Study the drawing (mm; zero at the part's minimum x, y, z) and answer. Coordinates: 2 decimals unless noted, no trailing zeros. Loops run counter-clockwise (first coordinate to the right, second up) from the corner with the lowest first, then second, coordinate; pieces in that order, holes last. Notation, with made-up numbers: (-9, 88.5) -> (4, 88.5) arc R14 cw to (4, 106.5) -> close; hole circle Ø5 at (59, 53.5). An arc over 180 degrees is marked (long way). Answer in a Markdown table with one row per item.
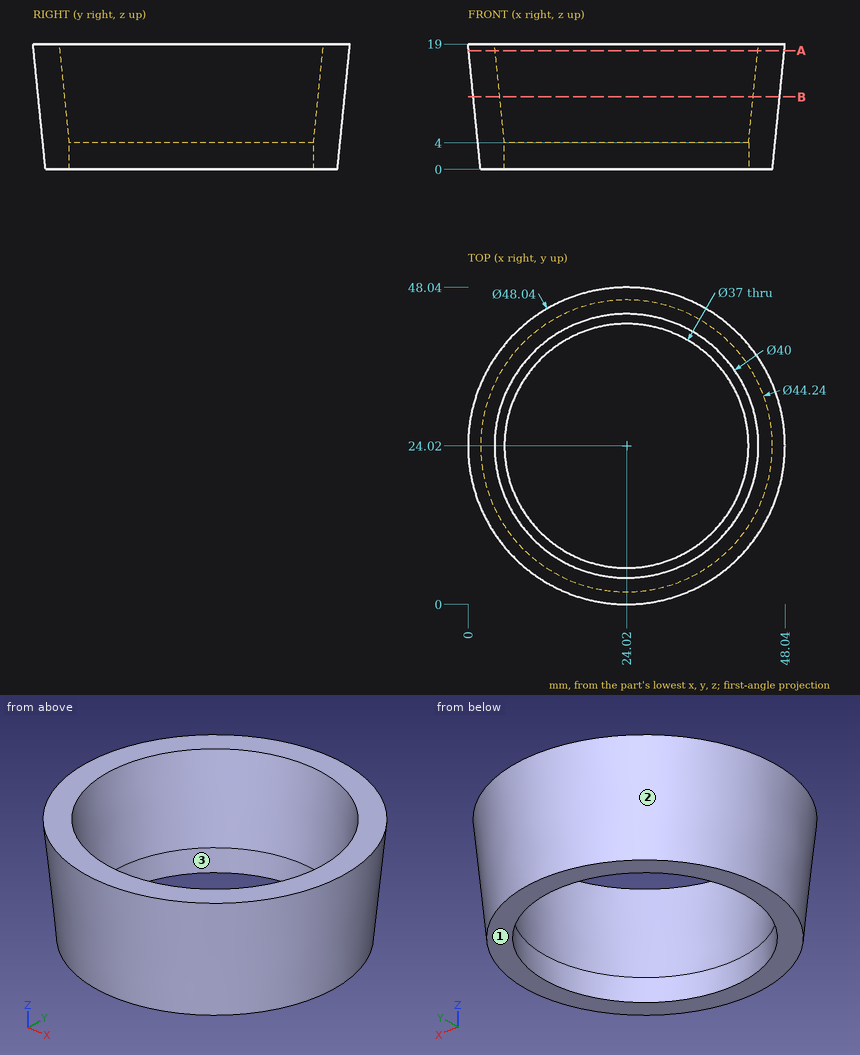
1. Find the intervals of material crossed by probe 1 along X at (y, z) = (26, 5.5); probe 2 along X at (y, z) = (15, 7.5); probe 3 along Y at (x, z) = (39.5, 11.25), in increasing order.
A:
| item | result |
|---|---|
| probe 1 | x = 1.44 to 5.48, 42.56 to 46.6 |
| probe 2 | x = 3 to 7.47, 40.57 to 45.04 |
| probe 3 | y = 6.68 to 12.62, 35.42 to 41.36 |
2. The mould has two halves that part along Y. Classify the marked faces 1, 2 and 3: pulls with the +Y half, pulls with the -Y half, needs draft (parallel to the pull), parting line crosses it, or undercut.
A:
| item | result |
|---|---|
| face 1 | needs draft |
| face 2 | parting line crosses it |
| face 3 | undercut |
3. Given pin 1 Ø4 at (y, z) = (6, 11.5) entering from +X; pin 2 Ø12 at (x, y) = (14.5, 30.5) entering from -Z; pin 3 Ø1.5 at (x, z) = (17, 9.5) entering from -Y; pin 4 Ø8 at (y, z) = (35, 14.5) entering from -X, each flat-ended and moving along its own axis, determine where each tip first touches the part or whether it passes through.
A:
| item | result |
|---|---|
| pin 1 | stops at x = 40.92 |
| pin 2 | passes through |
| pin 3 | stops at y = 1.8 |
| pin 4 | stops at x = 1.44 |
4. A cutting plane is placed at A-A on z = 18. Give the vertices of the cut face in (x, y).
A:
| item | result |
|---|---|
| outline | circle Ø47.84 at (24.02, 24.02); hole circle Ø39.8 at (24.02, 24.02) |
5. A cutting plane is placed at B-B on z = 11. Give the vertices of the cut face in (x, y), and give its area (3 significant figures).
A:
| item | result |
|---|---|
| outline | circle Ø46.44 at (24.02, 24.02); hole circle Ø38.4 at (24.02, 24.02) |
| area | 536 mm2 |
